Can you work these out from the model? Positions are in its coordinate system, mm. Face numbers are marked on the shaded views. A direction names the side the tool comes from. Give positions to 0.01 mm unless a question says otherwise; leave off trailing zeros. Order: outer loops, then holes, each group sorted by start corner. A loop starts at its lowest first (then second) coordinate and runs counter-clockwise, first axis right, second up. Notation, with made-up numbers: M 55.5,65.5 L 103.5,65.5 A30 cw 103.5,91.5 Z; hole C 49.25,61.5 d3. An arc over 180 degrees is marked long. Write each question's results on one line, items separated by ' | '.
from build123d import *

# Parameters (mm, degrees)
SKETCH_1_R          = 10
EXTRUDE_1_DEPTH     = 5
SKETCH_2_R          = 4.5
CUT_EXTRUDE_1_DEPTH = 3
CHAMFER_1_SIZE      = 2


with BuildPart() as part:
    # 草圖1 → 填料-伸長1 (new body)
    with BuildSketch(Plane(origin=(0, 0, 0), x_dir=(1, 0, 0), z_dir=(0, 1, 0))):
        with Locations(Location((0, 0, 0), (0, 0, 270))):
            Circle(SKETCH_1_R)
    extrude(amount=EXTRUDE_1_DEPTH)

    # 草圖2 → 除料-伸長1 (cut)
    with BuildSketch(Plane(origin=(0, 5, 0), x_dir=(1, 0, 0), z_dir=(0, 1, 0))):
        with Locations(Location((0, 0, 0), (0, 0, 270))):
            Circle(SKETCH_2_R)
    extrude(amount=-CUT_EXTRUDE_1_DEPTH, mode=Mode.SUBTRACT)

    # 導角1
    chamfer_1_edges = [part.edges().sort_by_distance(p)[0] for p in [
        (0, 0, -10),
    ]]
    chamfer(chamfer_1_edges, length=CHAMFER_1_SIZE)


solid = part.part
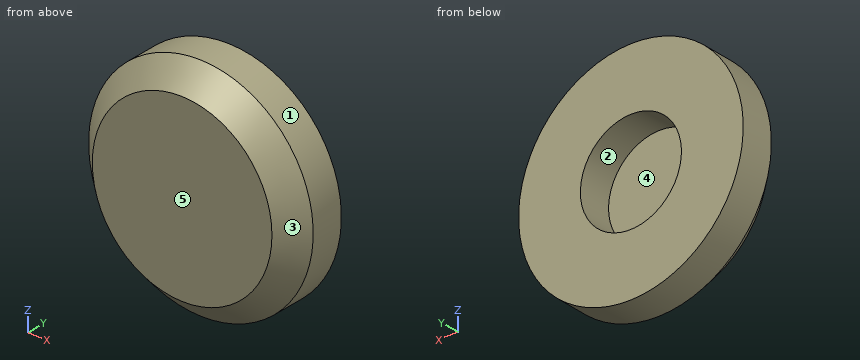
(1) Imagine slicing it at B-B, the plane z = 0. Write out the boundary of the cut face in (x, y), plus the area to 3 significant figures.
Data:
outline: M -10,2 L -8,0 L 8,0 L 10,2 L 10,5 L 4.5,5 L 4.5,2 L -4.5,2 L -4.5,5 L -10,5 Z | area: 69.0 mm2
(2) For the marked faces 1 and 2, which set-ups out of +Z, -Z, +X, -X, +Y, -Y let a thin tool reach every point of the face, with its end or its side?
Data:
face 1: +Y, -Y | face 2: +Y
(3) Imagine slicing it at A-A, the plane x = 0. Write out the boundary of the cut face in (y, z).
Data:
outline: M 0,-8 L 2,-10 L 5,-10 L 5,-4.5 L 2,-4.5 L 2,4.5 L 5,4.5 L 5,10 L 2,10 L 0,8 Z
(4) Will these pins go through, and if not, where does the flat tip stop? P1, Ø3, axis at x = 4, y = 2, coming from the -Z side; P2, Ø1, axis at x = -2.5, y = 4, coming from the +Z side.
Data:
P1: stops at z = -9.68 | P2: stops at z = 9.8
(5) I need wall thicknesses on L1, parallel to X at y = 3, z = 0; L2, parallel to Y at x = 3.5, z = 0; L3, parallel to Z at x = -0.25, y = 4.35. Which ranges of each line are inside material? Lowest first, please. Write a range as from..to.
Data:
L1: x = -10..-4.5, 4.5..10 | L2: y = 0..2 | L3: z = -10..-4.49, 4.49..10
(6) Imagine slicing it at C-C, the plane y = 2.5. Write out the boundary of the cut face in (x, z), plus the area to 3 significant figures.
Data:
outline: C 0,0 d20; hole C 0,0 d9 | area: 251 mm2
(7) We'd pull the mould along X, two halves only. Please class the marked faces 3, 4 and 5: +X half, -X half, draft (parallel to the pull), parting line (faces both ways), or undercut.
Data:
face 3: parting line | face 4: undercut | face 5: draft
(8) Imagine slicing it at D-D, the plane y = 1.1. Write out the boundary of the cut face in (x, z), plus the area to 3 significant figures.
Data:
outline: C 0,0 d18.2 | area: 260 mm2
